Here's how the part is built. I have some questions about the finished solid (model axes, mm). A direction names the side the tool comes from. Coordinates: 2 decimals unless noted, no trailing zeros. Write each loop counter-clockwise with the first axis right and the second up, starting at its lowest first coordinate (ties: lowest second). Pieces come first, ordered by that corner, then holes. Notation, with made-up numbers: M 9,16.5 L 14,16.5 A21 ccw 14,25.5 Z; hole C 85.25,5 d11. An arc over 180 degrees is marked long. Use a Markdown table: item, result.
```python
from build123d import *

# Parameters (mm, degrees)
RESSALTO_EXTRUS_O1_DEPTH = 48
ESBO_O12_R               = 1.5
CORTE_EXTRUS_O10_DEPTH   = 10
ESBO_O13_R               = 1.5
CORTE_EXTRUS_O11_DEPTH   = 10
ESBO_O14_R               = 1.5
CORTE_EXTRUS_O12_DEPTH   = 10
ESBO_O15_R               = 1.5
CORTE_EXTRUS_O13_DEPTH   = 10
CORTE_EXTRUS_O14_DEPTH   = 10
ESBO_O17_R               = 4
ESBO_O17_W               = 2.8
ESBO_O17_H               = 2.8
RESSALTO_EXTRUS_O2_DEPTH = 4
CORTE_EXTRUS_O15_DEPTH   = 10


with BuildPart() as part:
    # Model → Ressalto-extrusão1 (new body)
    with BuildSketch(Plane.XY):
        with BuildLine():
            Line((-0.7, 0), (39, 0))
            Line((39, 0), (39.7, 0))
            Line((39.7, 0), (39.7, -11.380317396))
            Line((39.7, -11.380317396), (50.182424304, -21.8627417))
            Line((50.182424304, -21.8627417), (58.119682605, -29.8))
            Line((58.119682605, -29.8), (81.7, -29.8))
            ThreePointArc((81.7, -29.8), (105.905643752, -13.626305928), (100.226197667, 14.926197667))
            Line((100.226197667, 14.926197667), (65.00338056, 50.149014774))
            Line((65.00338056, 50.149014774), (50.111140335, 50.149014774))
            Line((50.111140335, 50.149014774), (14.181595121, 50.149014774))
            Line((14.181595121, 50.149014774), (-3.2, 32.767419653))
            Line((-3.2, 32.767419653), (-3.2, 5))
            Line((-3.2, 5), (-3.2, 0))
            Line((-3.2, 0), (-0.7, 0))
        make_face()
        with BuildLine():
            Line((-0.7, 2.5), (39, 2.5))
            Line((39, 2.5), (39.7, 2.5))
            Line((39.7, 2.5), (42.2, 2.5))
            Line((42.2, 2.5), (42.2, -10.34478349))
            Line((42.2, -10.34478349), (51.950191257, -20.094974747))
            Line((51.950191257, -20.094974747), (59.15521651, -27.3))
            Line((59.15521651, -27.3), (81.7, -27.3))
            ThreePointArc((81.7, -27.3), (103.595944921, -12.669597347), (98.458430714, 13.158430714))
            Line((98.458430714, 13.158430714), (63.967846654, 47.649014774))
            Line((63.967846654, 47.649014774), (50.111140335, 47.649014774))
            Line((50.111140335, 47.649014774), (15.217129027, 47.649014774))
            Line((15.217129027, 47.649014774), (-0.7, 31.731885747))
            Line((-0.7, 31.731885747), (-0.7, 2.5))
        make_face(mode=Mode.SUBTRACT)
    extrude(amount=RESSALTO_EXTRUS_O1_DEPTH)

    # Esboço12 → Corte-extrusão10 (cut)
    with BuildSketch(Plane(origin=(57.576197667, 57.576197667, 0), x_dir=(0, 0, -1), z_dir=(0.7071067811865476, 0.7071067811865475, 0))):
        with Locations(Location((-44, -20.072657306, 0), (0, 0, 90))):
            Circle(ESBO_O12_R)
        with Locations(Location((-44, -52.072657306, 0), (0, 0, 90))):
            Circle(ESBO_O12_R)
    extrude(amount=-CORTE_EXTRUS_O10_DEPTH, mode=Mode.SUBTRACT)

    # Esboço13 → Corte-extrusão11 (cut)
    with BuildSketch(Plane(origin=(0, 50.149014774, 0), x_dir=(1, 0, 0), z_dir=(0, 1, 0))):
        with Locations(Location((39.59248784, -44, 0), (0, 0, 270))):
            Circle(ESBO_O13_R)
    extrude(amount=-CORTE_EXTRUS_O11_DEPTH, mode=Mode.SUBTRACT)

    # Esboço14 → Corte-extrusão12 (cut)
    with BuildSketch(Plane.ZY.offset(3.2)):
        with Locations((44, 23.701037279)):
            Circle(ESBO_O14_R)
        with Locations((44, 7.740898975)):
            Circle(ESBO_O14_R)
    extrude(amount=-CORTE_EXTRUS_O12_DEPTH, mode=Mode.SUBTRACT)

    # Esboço15 → Corte-extrusão13 (cut)
    with BuildSketch(Plane(origin=(14.159841302, 14.159841302, 0), x_dir=(0, 0, 1), z_dir=(-0.7071067811865477, -0.7071067811865475, 0))):
        with Locations(Location((44, -46.881179593, 0), (0, 0, 270))):
            Circle(ESBO_O15_R)
    extrude(amount=-CORTE_EXTRUS_O13_DEPTH, mode=Mode.SUBTRACT)

    # Esboço16 → Corte-extrusão14 (cut)
    with BuildSketch(Plane.XY.offset(48)):
        Polygon((39.7, 0), (39.7, -7.84478349), (42.2, -10.34478349), (42.2, 2.5), (-0.7, 2.5), (-0.7, 0), align=None)
    extrude(amount=-CORTE_EXTRUS_O14_DEPTH, mode=Mode.SUBTRACT)

    # Esboço17 → Ressalto-extrusão2 (add)
    # profile 1 of 6: a face of its own
    with BuildSketch(Plane(origin=(0, 0, 0), x_dir=(-1, 0, 0), z_dir=(0, 0, -1))):
        with Locations((-91.568699638, 17.926841447)):
            Circle(ESBO_O17_R)
        with Locations((-91.568699638, 17.926841447)):
            Rectangle(ESBO_O17_W, ESBO_O17_H, mode=Mode.SUBTRACT)
    # profile 2 of 6: a face of its own
    with BuildSketch(Plane(origin=(0, 0, 0), x_dir=(-1, 0, 0), z_dir=(0, 0, -1))):
        with Locations((-68.47265349, 41.022887595)):
            Circle(ESBO_O17_R)
        with Locations((-68.47265349, 41.022887595)):
            Rectangle(ESBO_O17_W, ESBO_O17_H, mode=Mode.SUBTRACT)
    # profile 3 of 6: a face of its own
    with BuildSketch(Plane(origin=(0, 0, 0), x_dir=(-1, 0, 0), z_dir=(0, 0, -1))):
        with Locations((-39.59248784, 46.149014774)):
            Circle(ESBO_O17_R)
        with Locations((-39.59248784, 46.149014774)):
            Rectangle(ESBO_O17_W, ESBO_O17_H, mode=Mode.SUBTRACT)
    # profile 4 of 6: a face of its own
    with BuildSketch(Plane(origin=(0, 0, 0), x_dir=(-1, 0, 0), z_dir=(0, 0, -1))):
        with Locations((-0.8, 24.383709827)):
            Circle(ESBO_O17_R)
        with Locations((-0.8, 24.383709827)):
            Rectangle(ESBO_O17_W, ESBO_O17_H, mode=Mode.SUBTRACT)
    # profile 5 of 6: a face of its own
    with BuildSketch(Plane(origin=(0, 0, 0), x_dir=(-1, 0, 0), z_dir=(0, 0, -1))):
        with Locations((-0.8, 8.383709827)):
            Circle(ESBO_O17_R)
        with Locations((-0.8, 8.383709827)):
            Rectangle(ESBO_O17_W, ESBO_O17_H, mode=Mode.SUBTRACT)
    # profile 6 of 6: a face of its own
    with BuildSketch(Plane(origin=(0, 0, 0), x_dir=(-1, 0, 0), z_dir=(0, 0, -1))):
        with Locations((-51.388268427, -17.411731573)):
            Circle(ESBO_O17_R)
        with Locations((-51.388268427, -17.411731573)):
            Rectangle(ESBO_O17_W, ESBO_O17_H, mode=Mode.SUBTRACT)
    extrude(amount=-RESSALTO_EXTRUS_O2_DEPTH)

    # Esboço18 → Corte-extrusão15 (cut)
    with BuildSketch(Plane.XY.offset(48)):
        Polygon((-0.7, 31.731885747), (-32.431885747, 0), (-0.7, 0), align=None)
    extrude(amount=-CORTE_EXTRUS_O15_DEPTH, mode=Mode.SUBTRACT)

    # Esboço19 → Corte-Revolução1 (revolve, cut)
    with BuildSketch(Plane.ZY.offset(3.2)):
        with BuildLine():
            Line((38.25689259, 0), (13.25689259, 0))
            Line((13.25689259, 0), (13.25689259, 3))
            ThreePointArc((13.25689259, 3), (14.721358684, 6.535533906), (18.25689259, 8))
            Line((18.25689259, 8), (38.25689259, 8))
            Line((38.25689259, 8), (38.25689259, 0))
        make_face()
    revolve(axis=Axis((-3.2, 0, 38.25689259), (0, 0, -1)), mode=Mode.SUBTRACT)


solid = part.part
```
1. Suppose I cut it at C-C on z = 23. Write out the boundary of the cut face in (x, y), and give its area (3 significant figures).
Answers follow:
| item | result |
|---|---|
| outline | M -3.2,8 A8 cw -0.7,7.6 L -0.7,31.73 L 15.22,47.65 L 63.97,47.65 L 98.46,13.16 A23.7 cw 81.7,-27.3 L 59.16,-27.3 L 42.2,-10.34 L 42.2,2.5 L 4.4,2.5 A8 cw 4.8,0 L 39.7,0 L 39.7,-11.38 L 58.12,-29.8 L 81.7,-29.8 A26.2 ccw 100.23,14.93 L 65,50.15 L 14.18,50.15 L -3.2,32.77 Z |
| area | 756 mm2 |
2. Which directions (+Z, -Z, +X, -X, +Y, -Y) give clear straight access to the entire face, cutting with the end or side of a thin tool? Please do faces 4 (the face through (3, 24, 4)), 5 (the face through (1, 9.784, 2)), 6 (the face through (39.7, -6, 18)).
Answers follow:
| item | result |
|---|---|
| face 4 | +Z |
| face 5 | +Z, -Z |
| face 6 | +Z, -Z, -X, -Y |
3. Will these pins go through, and if not, where does the flat tip stop? pin 1 Ø9 at (y, z) = (-7, 25) entering from -X; pin 2 Ø8 at (x, z) = (12.5, 6) entering from -Y; pin 3 Ø2 at (x, z) = (40, 1.5) entering from -Y; pin 4 Ø10 at (y, z) = (19, 40) entering from -X.
Answers follow:
| item | result |
|---|---|
| pin 1 | stops at x = 39.7 |
| pin 2 | stops at y = 0 |
| pin 3 | stops at y = -12.68 |
| pin 4 | stops at x = -3.2 |
4. Suppose I cut it at D-D on z = 44. State how many separate pieces and enclosed holes the cut face has, and give its area (3 significant figures).
Answers follow:
| item | result |
|---|---|
| separate pieces | 5 |
| enclosed holes | 0 |
| area | 553 mm2 |
5. Suppose I cut it at A-A on z = 8.5. Write out the boundary of the cut face in (x, y).
Answers follow:
| item | result |
|---|---|
| outline | M -3.2,0 L 39.7,0 L 39.7,-11.38 L 58.12,-29.8 L 81.7,-29.8 A26.2 ccw 100.23,14.93 L 65,50.15 L 14.18,50.15 L -3.2,32.77 Z; hole M -0.7,2.5 L 42.2,2.5 L 42.2,-10.34 L 59.16,-27.3 L 81.7,-27.3 A23.7 ccw 98.46,13.16 L 63.97,47.65 L 15.22,47.65 L -0.7,31.73 Z |
6. We'd pull the mould along X, two halves only. Please class faces 1 (the face through (2.2, 8, 2)), 2 (the face through (81, 31, 48)), 3 (the face through (105.74, -14.02, 23.66)): +X half, -X half, draft (parallel to the pull), parting line (faces both ways), or undercut.
Answers follow:
| item | result |
|---|---|
| face 1 | undercut |
| face 2 | draft |
| face 3 | +X half |
7. I need wall thicknesses on probe 1 along Y at (x, z) = (24, 28.5); probe 2 along Y at (x, z) = (47.5, 25); probe 3 along X at (y, z) = (-4, 35). Which ranges of each line are inside material? Lowest first, please.
Answers follow:
| item | result |
|---|---|
| probe 1 | y = 0 to 2.5, 47.65 to 50.15 |
| probe 2 | y = -19.18 to -15.64, 47.65 to 50.15 |
| probe 3 | x = 39.7 to 42.2, 105.4 to 107.9 |
8. Suppose I cut it at B-B on x = 8.5. Write out the boundary of the cut face in (y, z), and give its area (3 significant figures).
Answers follow:
| item | result |
|---|---|
| outline | M 0,0 L 2.5,0 L 2.5,38 L 0,38 Z; M 40.93,0 L 44.47,0 L 44.47,48 L 40.93,48 Z |
| area | 265 mm2 |
